Design review of the part shown in the three views and the two pictorial views. Dimensions are in mm from the part's minimum x, y and z. A direction names the side the tool comes from. Round coordinates to 2 decimals unless told otherwise and drop trailing zeros. Order: outer loops, then holes, each group sorted by start corner. A loop starts at its lowest first (then second) coordinate and runs counter-clockwise, first axis right, second up.
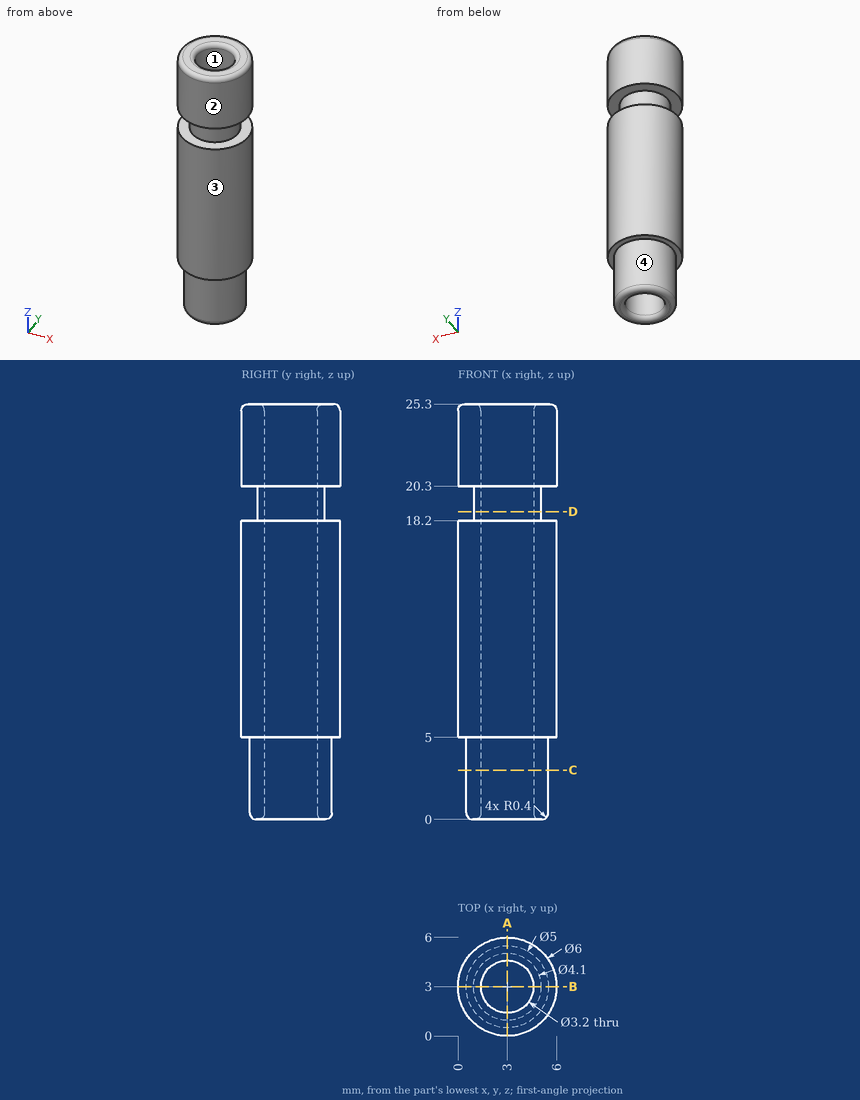
1) The part is to be moulded in two halves that separate along X. For the marked faces 1 and 2, say which applies: released by +X, released by -X, zero draft, split by the parting line, or undercut.
Results:
face 1: undercut
face 2: split by the parting line
2) Take a section at D-D on z = 18.75. Give the boundary of the cut face in (x, y), plus the area to 3 significant figures.
Results:
outline: circle Ø4.1 at (3, 3); hole circle Ø3.2 at (3, 3)
area: 5.16 mm2
3) For the marked faces 3 and 4, list the 3-axis set-ups (+Z, -Z, +X, -X, +Y, -Y) from which the entire face can be reached by the end or side of a thin tool; tool diameter is ignored.
Results:
face 3: +Z, -Z
face 4: -Z
4) Take a section at A-A on x = 3. Give the boundary of the cut face in (y, z), plus the area to 3 significant figures.
Results:
outline: (0, 5) - (0.5, 5) - (0.5, 0.4) arc R0.4 ccw to (0.9, 0) - (1, 0) arc R0.4 ccw to (1.4, 0.4) - (1.4, 24.9) arc R0.4 ccw to (1, 25.3) - (0.4, 25.3) arc R0.4 ccw to (0, 24.9) - (0, 20.3) - (0.95, 20.3) - (0.95, 18.2) - (0, 18.2) - close; (4.6, 0.4) arc R0.4 ccw to (5, 0) - (5.1, 0) arc R0.4 ccw to (5.5, 0.4) - (5.5, 5) - (6, 5) - (6, 18.2) - (5.05, 18.2) - (5.05, 20.3) - (6, 20.3) - (6, 24.9) arc R0.4 ccw to (5.6, 25.3) - (5, 25.3) arc R0.4 ccw to (4.6, 24.9) - close
area: 61.6 mm2
5) Clearance check with flat-ended pins moving along their axes: P1, Ø2, axis at x = 1.5, z = 11.5, coming from the -Y side; P2, Ø1.5, axis at y = 3, z = 2.5, coming from the +X side; P3, Ø3, axis at y = 3, z = 19.5, coming from the -X side. State where each tip first meets the part, or that it passes through.
Results:
P1: stops at y = 0.04
P2: stops at x = 5.5
P3: stops at x = 0
6) To check wall thickness, follow line 1 along Y through (x, z) = (3, 16.25); line 2 along Z through (x, y) = (1.7, 0.8). State the ranges of each line that lie inside material, in increasing order.
Results:
line 1: y = 0 to 1.4, 4.6 to 6
line 2: z = 5 to 18.2, 20.3 to 25.3
7) Take a section at C-C on z = 3. Give the boundary of the cut face in (x, y), plus the area to 3 significant figures.
Results:
outline: circle Ø5 at (3, 3); hole circle Ø3.2 at (3, 3)
area: 11.6 mm2
